```python
from build123d import *

# Parameters (mm, degrees)
SKETCH_5_W          = 25.4
SKETCH_5_H          = 25.4
SKETCH_5_W_2        = 19.05
SKETCH_5_H_2        = 19.05
EXTRUDE_1_DEPTH     = 25.4
SKETCH_6_R          = 1.5875
CUT_EXTRUDE_1_DEPTH = 30.48
SKETCH_7_R          = 1.5875
CUT_EXTRUDE_2_DEPTH = 30.48


with BuildPart() as part:
    # 스케치5 → 보스-돌출1 (new body)
    with BuildSketch(Plane(origin=(0, 0, 0), x_dir=(1, 0, 0), z_dir=(0, 1, 0))):
        Rectangle(SKETCH_5_W, SKETCH_5_H)
        Rectangle(SKETCH_5_W_2, SKETCH_5_H_2, mode=Mode.SUBTRACT)
    extrude(amount=EXTRUDE_1_DEPTH)

    # 스케치6 → 컷-돌출1 (cut)
    with BuildSketch(Plane.XY.offset(12.7)):
        with Locations((0, 12.7)):
            Circle(SKETCH_6_R)
    extrude(amount=-CUT_EXTRUDE_1_DEPTH, mode=Mode.SUBTRACT)

    # 스케치7 → 컷-돌출2 (cut)
    with BuildSketch(Plane(origin=(12.7, 0, 0), x_dir=(0, 0, -1), z_dir=(1, 0, 0))):
        with Locations((0, 12.7)):
            Circle(SKETCH_7_R)
    extrude(amount=-CUT_EXTRUDE_2_DEPTH, mode=Mode.SUBTRACT)


solid = part.part
```
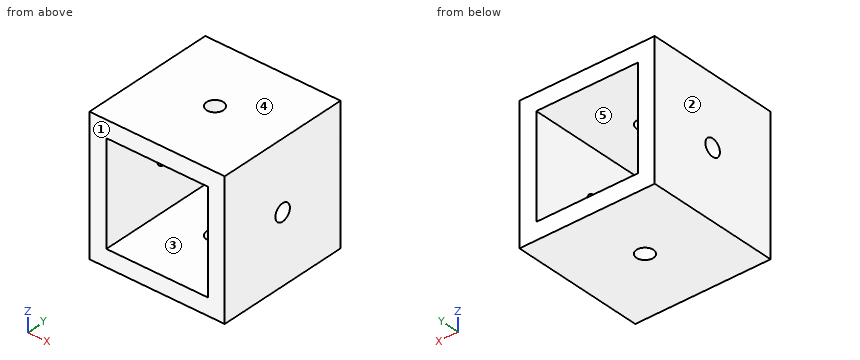
Here's how the part is built. I have some questions about the finished solid (model axes, mm). Face numbers are marked on the shaded views. A direction names the side the tool comes from. Give positions to 0.01 mm unless a question says otherwise; leave off trailing zeros. Order: outer loops, then holes, each group sorted by start corner. A loop starts at its lowest first (then second) coordinate and runs counter-clockwise, first axis right, second up. Notation, with made-up numbers: M 55,39 L 98,39 A21 cw 98,43 Z; hole C -35,36.25 d7. An arc over 180 degrees is marked long. Use a Markdown table: item, result. Add a question column.
1. On a 3-axis mill with a long thin cutter (end or side, diameter ignored), from which of +Z, -Z, +X, -X, +Y, -Y can I reach the whole of each face in a straight line? I mean the marked faces 4 and 5. Say none if no direction works.
2. Suppose I cut it at A-A (z = 2.5). List the corners of the cut face in (x, y) for me (3 decimals).
3. Suppose I cut it at C-C (y = 12.7). List the corners of the cut face in (x, z) for me (1 decimal).
4. Suppose I cut it at D-D (x = 0). List the corners of the cut face in (y, z) for me (1 decimal), and give its area (3 significant figures).
5. For pin 1 Ø5 at (y, z) = (12.7, 0) entering from -X; pin 2 Ø2.5 at (y, z) = (12.7, 0) entering from -X, each with a flat end and sliding along its axis, tell me the tip position at first contact or that it passes through.
6. I need wall thicknesses on probe 1 along Z at (x, y) = (-1, 19) (3 decimals); probe 2 along Y at (x, z) = (11.6, 0). Which ranges of each line are inside material? Lowest first, please. Write a range as from..to.
7. If we mould it in two halves opening along X, with no side actions, what happens to the marked faces 1, 2 and 3? For each: +X half, -X half, draft (parallel to the pull), parting line (faces both ways), or undercut.
8. Suppose I cut it at B-B (x = -4.5). List the corners of the cut face in (y, z) for me (3 decimals), and give its area (3 significant figures).
Results list:
| question | item | result |
|---|---|---|
| 1 | face 4 | +Z, +X, -X, +Y, -Y |
| 1 | face 5 | +Y, -Y |
| 2 | outline | M -12.7,0 L -9.525,0 L -9.525,25.4 L -12.7,25.4 Z; M 9.525,0 L 12.7,0 L 12.7,25.4 L 9.525,25.4 Z |
| 3 | outline | M -12.7,-12.7 L -1.6,-12.7 L -1.6,-9.5 L -9.5,-9.5 L -9.5,-1.6 L -12.7,-1.6 Z; M -12.7,1.6 L -9.5,1.6 L -9.5,9.5 L -1.6,9.5 L -1.6,12.7 L -12.7,12.7 Z; M 1.6,-12.7 L 12.7,-12.7 L 12.7,-1.6 L 9.5,-1.6 L 9.5,-9.5 L 1.6,-9.5 Z; M 1.6,9.5 L 9.5,9.5 L 9.5,1.6 L 12.7,1.6 L 12.7,12.7 L 1.6,12.7 Z |
| 4 | outline | M 0,-12.7 L 11.1,-12.7 L 11.1,-9.5 L 0,-9.5 Z; M 0,9.5 L 11.1,9.5 L 11.1,12.7 L 0,12.7 Z; M 14.3,-12.7 L 25.4,-12.7 L 25.4,-9.5 L 14.3,-9.5 Z; M 14.3,9.5 L 25.4,9.5 L 25.4,12.7 L 14.3,12.7 Z |
| 4 | area | 141 mm² |
| 5 | pin 1 | stops at x = -12.7 |
| 5 | pin 2 | passes through |
| 6 | probe 1 | z = -12.7..-9.525, 9.525..12.7 |
| 6 | probe 2 | y = 0..11.11, 14.29..25.4 |
| 7 | face 1 | draft |
| 7 | face 2 | -X half |
| 7 | face 3 | undercut |
| 8 | outline | M 0,-12.7 L 25.4,-12.7 L 25.4,-9.525 L 0,-9.525 Z; M 0,9.525 L 25.4,9.525 L 25.4,12.7 L 0,12.7 Z |
| 8 | area | 161 mm² |
